Input: part model. Units: mm. Frame: model coordinates. A direction names the side the tool comes from. Give positions to 0.01 mm unless a question says otherwise; leave off trailing zeros. Write each loop counter-clockwise with the first axis right and the second up, starting at its lowest first coordinate (ties: lowest second). Pieces come first, ordered by that corner, then holes.
```python
from build123d import *

# Parameters (mm, degrees)
SKETCH1_R           = 6.35
BOSS_EXTRUDE1_DEPTH = 1.5875
SKETCH2_W           = 2.1
SKETCH2_H           = 3.175
CUT_EXTRUDE1_DEPTH  = 10.119493201


with BuildPart() as part:
    # Sketch1 → Boss-Extrude1 (new body)
    with BuildSketch(Plane.XY):
        Circle(SKETCH1_R)
        Polygon((-3.175, -1.5875), (-3.175, 1.5875), (-1.5875, 1.5875), (-1.5875, 3.175), (1.5875, 3.175), (1.5875, 1.5875), (3.175, 1.5875), (3.175, -1.5875), (1.5875, -1.5875), (1.5875, -3.175), (-1.5875, -3.175), (-1.5875, -1.5875), align=None, mode=Mode.SUBTRACT)
    extrude(amount=BOSS_EXTRUDE1_DEPTH)

    # Sketch2 → Cut-Extrude1 (cut, through all)
    with BuildSketch(Plane(origin=(0, 0, 0), x_dir=(-1, 0, 0), z_dir=(0, 0, -1))):
        with Locations((0, -4.7625)):
            Rectangle(SKETCH2_W, SKETCH2_H)
    extrude(amount=-CUT_EXTRUDE1_DEPTH, mode=Mode.SUBTRACT)


solid = part.part
```
Item 1: Pin query (flat end, axial travel): pin 1 (1.5 mm diameter, centred on x = 1, y = 3, fed in from -Z); pin 2 (0.8 mm diameter, centred on y = 2.5, z = 0.5, fed in from +X); pin 3 (0.8 mm diameter, centred on x = 0.5, z = 1, fed in from -Y) (3 decimals); pin 4 (0.8 mm diameter, centred on y = -2, z = 0.5, fed in from -X). Return the tip coordinate at first contact, or that it passes through.
Item 2: Mould query, pull axis Y, two halves, no side actions, for faces 4 (the flat face through (-1.05, -5, 1)), 5 (the flat face through (2, 1.588, 1)), 6 (the cylindrical face through (0.264, 6.344, 0.783)). Classes: +Y half, -Y half, draft (parallel to the pull), parting line (faces both ways), or undercut.
Item 3: Section B-B (x = -3). Return loops of the section in (y, z).
Item 4: Ray query, line 1 (X direction, y = 0.25, z = 0.9) (3 decimals); line 2 (X direction, y = -3, z = 1.4); line 3 (Y direction, x = -1.5, z = 1.3) (3 decimals). Return the intervals inside material, ascending.
Item 5: Set-up query: faces 1 (the flat face through (1.05, -5, 1)), 2 (the flat face through (3, -3, 0)), 3 (the flat face through (-1.588, 2, 1)). Return all of +Z, -Z, +X, -X, +Y, -Y with unobstructed straight access to the full face (end or side cutting, diameter ignored); none if empty.
Solved:
1. pin 1: stops at z = 0
1. pin 2: stops at x = 5.99
1. pin 3: stops at y = 3.175
1. pin 4: stops at x = -6.15
2. face 4: draft
2. face 5: undercut
2. face 6: parting line
3. outline: (-5.6, 0) - (-1.59, 0) - (-1.59, 1.59) - (-5.6, 1.59) - close; (1.59, 0) - (5.6, 0) - (5.6, 1.59) - (1.59, 1.59) - close
4. line 1: x = -6.345 to -3.175, 3.175 to 6.345
4. line 2: x = -5.6 to -1.59, 1.59 to 5.6
4. line 3: y = -6.17 to -3.175, 3.175 to 6.17
5. face 1: +Z, -Z, -Y
5. face 2: -Z, +X, -X, +Y, -Y
5. face 3: +Z, -Z
